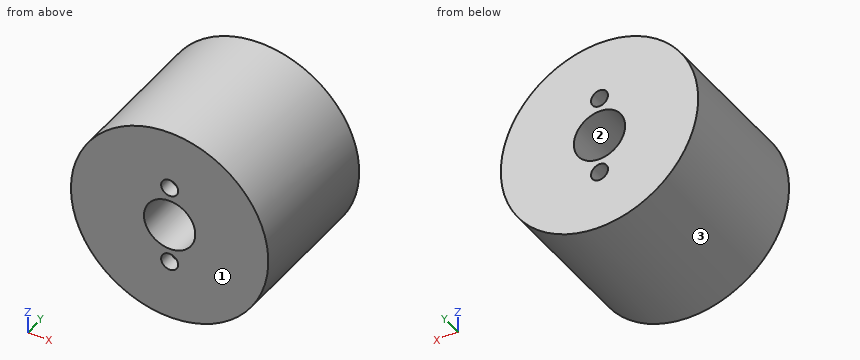
Autodesk Inventor part; units mm, degrees
ref_plane "YZ Plane" through (0, 0, 0) normal (1, 0, 0) x (0, 1, 0)
ref_plane "XZ Plane" through (0, 0, 0) normal (0, 1, 0) x (-1, 0, 0)
ref_plane "XY Plane" through (0, 0, 0) normal (0, 0, 1) x (1, 0, 0)
sketch "Sketch1" plane through (0, 0, 0) normal (0, 1, 0) x (-1, 0, 0)
  circle A0 centre (0, 0) radius 12.7
  circle A1 centre (0, 0) radius 3.302
  dimension "d0" = 25.4
  dimension "d1" = 6.604
extrude "Extrusion1" add sketch "Sketch1" along normal blind 19.05
sketch "Sketch2" plane through (0, 19.05, 0) normal (0, 1, 0) x (1, 0, 0)
  line L0 (0, 0) -> (0, -5.08)
  line L1 (0, -5.08) -> (0, 0)
  line L2 (0, 0) -> (0, 5.08)
  circle A0 centre (0, -5.08) radius 1.0922
  circle A1 centre (0, 5.08) radius 1.0922
  dimension "d4" = 5.08
  dimension "d5" = 5.08
  dimension "d6" = 2.1844
  dimension "d7" = 2.1844
extrude "Extrusion2" cut sketch "Sketch2" against normal blind 4.445
sketch "Sketch3" plane through (0, 0, 0) normal (0, -1, 0) x (1, 0, 0)
  line L0 (0, 0) -> (0, 5.08)
  line L1 (0, 5.08) -> (0, -5.08)
  circle A0 centre (0, 5.08) radius 1.0922
  circle A1 centre (0, -5.08) radius 1.0922
  dimension "d10" = 5.08
  dimension "d11" = 10.16
  dimension "d14" = 2.1844
  dimension "d15" = 2.1844
extrude "Extrusion3" cut sketch "Sketch3" against normal blind 1.905
properties part number "45DegreeMirrorPost_0p75in"
Geometry: final body of the model. Coordinates: model frame, mm. Face numbers are marked on the shaded views. Give positions to 0.01 mm unless a question says otherwise; leave off trailing zeros. Loops run counter-clockwise (first coordinate to the right, second up) from the corner with the lowest first, then second, coordinate; pieces in that order, holes last. Notation, with made-up numbers: (28.25, -38.5) - (42.25, -38.5) arc R20 ccw to (42.25, -15.5) - close; hole circle Ø6 at (8, 31.25). An arc over 180 degrees is marked (long way). Answer as CSV lines item,"result". Start each with the question number.
1. Ray query, L1, parallel to Z at x = 0, y = 1; L2, parallel to X at y = 15.95, z = 5.08; L3, parallel to X at y = 1, z = -1. Return the intervals inside material, ascending.
2. Section D-D, the plane z = 5.08. Return loops of the section in (x, y) (3 decimals).
3. Section C-C, the plane y = 2.75. Return loops of the section in (x, z), plus the area to 3 significant figures.
4. Section A-A, the plane x = 0. Return loops of the section in (y, z) (3 decimals), plus the area to 3 significant figures.
5. Pin query (flat end, axial travel): P1, Ø6, axis at y = 10.5, z = -6, coming from the -X side; P2, Ø1.1, axis at x = 0.5, z = -5, coming from the +Y side (3 decimals); P3, Ø1.5, axis at x = 1.5, y = 15.5, coming from the +Z side; P4, Ø2.5, axis at x = -0.5, z = 5.5, coming from the +Y side. Return the tip coordinate at first contact, or that it passes through.
6. Draft query along X for the marked faces 1, 2 and 3. Return one class per face: released by +X, released by -X, zero draft, split by the parting line, or undercut.
7. Section B-B, the plane z = -0.75. Return loops of the section in (x, y), plus the area to 3 significant figures.
Answers:
1,L1,"z = -12.7 to -6.17, -3.99 to -3.3, 3.3 to 3.99, 6.17 to 12.7"
1,L2,"x = -11.64 to -1.09, 1.09 to 11.64"
1,L3,"x = -12.66 to -3.15, 3.15 to 12.66"
2,outline,"(-11.64, 0) - (-1.092, 0) - (-1.092, 1.905) - (1.092, 1.905) - (1.092, 0) - (11.64, 0) - (11.64, 19.05) - (1.092, 19.05) - (1.092, 14.605) - (-1.092, 14.605) - (-1.092, 19.05) - (-11.64, 19.05) - close"
3,outline,"circle Ø25.4 at (0, 0); hole circle Ø6.6 at (0, 0)"
3,area,"472 mm2"
4,outline,"(0, -12.7) - (19.05, -12.7) - (19.05, -6.172) - (14.605, -6.172) - (14.605, -3.988) - (19.05, -3.988) - (19.05, -3.302) - (0, -3.302) - (0, -3.988) - (1.905, -3.988) - (1.905, -6.172) - (0, -6.172) - close; (0, 3.302) - (19.05, 3.302) - (19.05, 3.988) - (14.605, 3.988) - (14.605, 6.172) - (19.05, 6.172) - (19.05, 12.7) - (0, 12.7) - (0, 6.172) - (1.905, 6.172) - (1.905, 3.988) - (0, 3.988) - close"
4,area,"330 mm2"
5,P1,"stops at x = -12.34"
5,P2,"stops at y = 14.605"
5,P3,"stops at z = 12.68"
5,P4,"stops at y = 19.05"
6,face 1,"zero draft"
6,face 2,"undercut"
6,face 3,"split by the parting line"
7,outline,"(-12.68, 0) - (-3.22, 0) - (-3.22, 19.05) - (-12.68, 19.05) - close; (3.22, 0) - (12.68, 0) - (12.68, 19.05) - (3.22, 19.05) - close"
7,area,"361 mm2"
